Input: part model. Units: mm. Frame: model coordinates. A direction names the side the tool comes from. Coordinates: 2 decimals unless noted, no trailing zeros. Loops run counter-clockwise (first coordinate to the right, second up) from the corner with the lowest first, then second, coordinate; pieces in that order, holes last.
(1) Section C-C, the plane x = 96.5. Return loops of the section in (y, z) (3 decimals), then the cut area to 3 significant figures.
(2) Section A-A, the plane y = 2.1. Give the number of separate pieces and of enclosed holes in the cut face, then the cut area to 3 significant figures.
(3) Contact query for flat-ended pins moving along their axis: P1, Ø2.5, axis at x = 0, z = -31.75, coming from the +Y side; P2, Ø1.5, axis at x = 60.5, y = 2, coming from the +Z side. Output: stop coordinate, or through.
(4) Set-up query: faces 4 (the face through (2, 0, 26)), 5 (the face through (17.61, 1.61, -67.488)). Return all of +Z, -Z, +X, -X, +Y, -Y with unobstructed straight access to the full face (end or side cutting, diameter ignored); none if empty.
(5) Section B-B, the plane z = 91.5. Return loops of the section in (x, y) (3 decimals), then the cut area to 3 significant figures.
(6) Line query: L1, parallel to Z at x = -0.5, y = 2.8; L2, parallel to Z at x = 31.75, y = 2.45; L3, parallel to Z at x = 55, y = 0.55. Output: solid intervals per line, ascending.
(7) Mould query, pull axis Z, two halves, no side actions, for faces 1 (the face through (-123.98, 1.57, -27.53)), 2 (the face through (2, 3.175, 26)), 3 (the face through (-3.86, 1.61, -5.04)). Classes: released by +Z, released by -Z, zero draft, split by the parting line, or undercut.
```python
from build123d import *

# Parameters (mm, degrees)
SKETCH1_R           = 127
BOSS_EXTRUDE1_DEPTH = 3.175
SKETCH2_R           = 6.35
CUT_EXTRUDE1_DEPTH  = 180.63318353
CUT_EXTRUDE2_DEPTH  = 180.63318353
SKETCH4_R           = 1.5875
CUT_EXTRUDE3_DEPTH  = 180.63318353
CIRPATTERN1_COUNT   = 4
FILLET1_R           = 2.54
SKETCH5_R           = 1.5875
CUT_EXTRUDE4_DEPTH  = 180.63318353


with BuildPart() as part:
    # Sketch1 → Boss-Extrude1 (new body)
    with BuildSketch(Plane(origin=(0, 0, 0), x_dir=(1, 0, 0), z_dir=(0, 1, 0))):
        with Locations(Location((0, 0, 0), (0, 0, 270))):
            Circle(SKETCH1_R)
    extrude(amount=BOSS_EXTRUDE1_DEPTH)

    # Sketch2 → Cut-Extrude1 (cut, through all)
    with BuildSketch(Plane(origin=(0, 3.175, 0), x_dir=(1, 0, 0), z_dir=(0, 1, 0))):
        with Locations(Location((0, 0, 0), (0, 0, 270))):
            Circle(SKETCH2_R)
    extrude(amount=-CUT_EXTRUDE1_DEPTH, mode=Mode.SUBTRACT)

    # Sketch3 → Cut-Extrude2 (cut, through all)
    with BuildSketch(Plane(origin=(0, 3.175, 0), x_dir=(1, 0, 0), z_dir=(0, 1, 0))):
        with BuildLine():
            Line((-0.69608151, 69.707591228), (-1.204718825, 120.643985149))
            ThreePointArc((-1.204718825, 120.643985149), (30.046443244, 116.817986877), (59.221085226, 104.981025331))
            Line((59.221085226, 104.981025331), (34.319233166, 60.837593106))
            ThreePointArc((34.319233166, 60.837593106), (17.387075213, 67.544440681), (-0.69608151, 69.707591228))
        make_face()
    extrude(amount=-CUT_EXTRUDE2_DEPTH, mode=Mode.SUBTRACT)

    # Sketch4 → Cut-Extrude3 (cut, through all)
    with BuildSketch(Plane(origin=(0, 3.175, 0), x_dir=(1, 0, 0), z_dir=(0, 1, 0))):
        with Locations(Location((0, -31.75, 0), (0, 0, 270))):
            Circle(SKETCH4_R)
    cut_extrude3 = extrude(amount=-CUT_EXTRUDE3_DEPTH, mode=Mode.SUBTRACT)

    # CirPattern1: Cut-Extrude3 ×4 about axis
    cirpattern1_axis = Axis((0, 0, 0), (0, 1, 0))
    for i in range(1, CIRPATTERN1_COUNT):
        add(cut_extrude3.rotate(cirpattern1_axis, i * 360 / CIRPATTERN1_COUNT), mode=Mode.SUBTRACT)

    # Fillet1
    fillet1_edges = [part.edges().sort_by_distance(p)[0] for p in [
        (34.319233166, 1.5875, -60.837593106),
        (-0.69608151, 1.5875, -69.707591228),
        (-1.204718825, 1.5875, -120.643985149),
        (59.221085226, 1.5875, -104.981025331),
    ]]
    fillet(fillet1_edges, radius=FILLET1_R)

    # Sketch5 → Cut-Extrude4 (cut, through all)
    with BuildSketch(Plane.XZ):
        with Locations(Location((89.061954982, 49.824926956, 0), (0, 0, 270))):
            Circle(SKETCH5_R)
        with Locations(Location((101.542683253, 0.581943478, 0), (0, 0, 90))):
            Circle(SKETCH5_R)
    extrude(amount=-CUT_EXTRUDE4_DEPTH, mode=Mode.SUBTRACT)


solid = part.part
```
Report:
1. outline: (0, -82.564) - (3.175, -82.564) - (3.175, 82.564) - (0, 82.564) - close
1. area: 524 mm2
2. separate pieces: 1
2. enclosed holes: 8
2. area: 48,000 mm2
3. P1: passes through
3. P2: stops at z = 112.07
4. face 4: +Z, -Z, +X, -X, -Y
4. face 5: +Y, -Y
5. outline: (-88.072, 0) - (88.072, 0) - (88.072, 3.175) - (-88.072, 3.175) - close
5. area: 559 mm2
6. L1: z = -127 to -119.83, -71.19 to -33.26, -30.24 to -6.33, 6.33 to 30.24, 33.26 to 127
6. L2: z = -122.97 to -116.36, -62.19 to -1.59, 1.59 to 122.97
6. L3: z = -114.47 to -107.27, -97.5 to 114.47
7. face 1: split by the parting line
7. face 2: zero draft
7. face 3: undercut
